Design review of the part shown in the three views and the two pictorial views. Dimensions are in mm from the part's minimum x, y and z. A direction names the side the tool comes from. Give positions to 0.01 mm unless a question says otherwise; leave off trailing zeros. Loops run counter-clockwise (first coordinate to the right, second up) from the corner with the lowest first, then second, coordinate; pieces in that order, holes last. Notation, with made-up numbers: (26.25, 1.25) - (37.25, 1.25) arc R25 ccw to (37.25, 21.25) - close; hole circle Ø7 at (34, 52). An arc over 180 degrees is marked (long way). Answer as a JSON object with one key per item and string values.
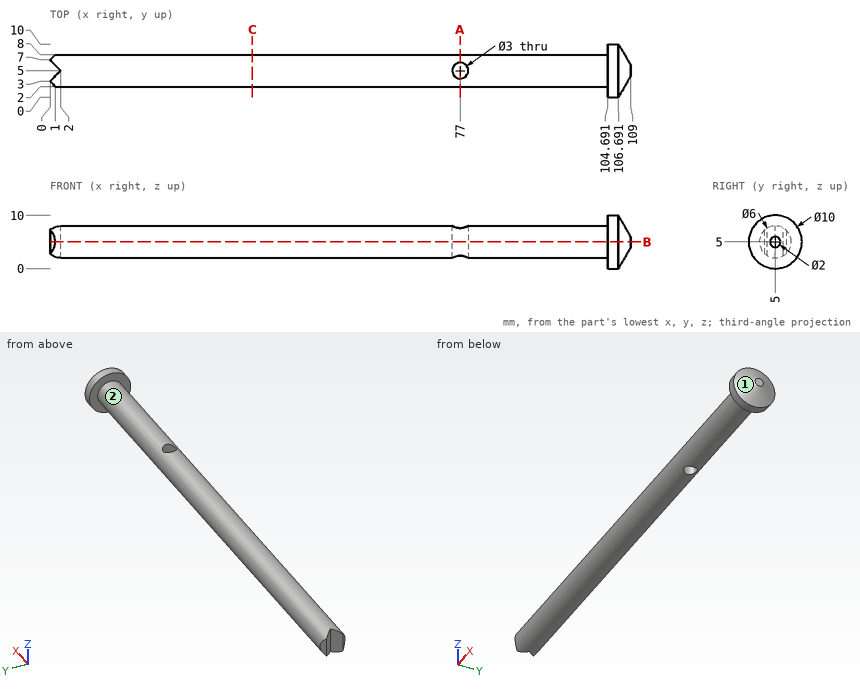
Q1. Clearance check with flat-ended pins moving along their axes: pin 1 Ø3 at (x, y) = (15.5, 8.5) entering from +Z (1 decimal); pin 2 Ø6 at (x, z) = (24, 8) entering from +Y; pin 3 Ø6 at (x, y) = (70, 2) entering from -Z; pin 4 Ø4 at (y, z) = (4, 3) entering from -X. State where each tip first meets the part, or that it passes through.
Results:
{"pin 1": "stops at z = 7.2", "pin 2": "stops at y = 8", "pin 3": "stops at z = 2", "pin 4": "stops at x = 0"}
Q2. Consider section A-A, the plane x = 77. State the section outline as (y, z) points.
Results:
{"outline": "(3.5, 2.4) - (3.5, 7.6) arc R3 ccw to start; (6.5, 2.4) arc R3 ccw to (6.5, 7.6) - close"}
Q3. For the marked faces 1 and 2, list the 3-axis set-ups (+Z, -Z, +X, -X, +Y, -Y) from which the entire face can be reached by the end or side of a thin tool; tool diameter is ignored.
Results:
{"face 1": "+X", "face 2": "-X"}
Q4. Consider section C-C, the plane x = 38. State the section outline as (y, z) points.
Results:
{"outline": "circle Ø6 at (5, 5)"}
Q5. Consider section B-B, the plane z = 5. State the section outline as (x, y) points, plus the area to 3 significant figures.
Results:
{"outline": "(0, 3) - (1, 2) - (104.69, 2) - (104.69, 0) - (106.69, 0) - (109, 4) - (109, 6) - (106.69, 10) - (104.69, 10) - (104.69, 8) - (1, 8) - (0, 7) - (2, 5) - close; hole circle Ø3 at (77, 5)", "area": "650 mm^2"}
Q6. To check wall thickness, follow probe 1 along X at (y, z) = (5, 5); probe 2 along Y at (x, z) = (57, 3) (1 decimal); probe 3 along Y at (x, z) = (77.5, 3.75) (1 decimal). State the ranges of each line that lie inside material, in increasing order. Write a range as [from, to].
Results:
{"probe 1": "x = [2, 75.5], [78.5, 109]", "probe 2": "y = [2.8, 7.2]", "probe 3": "y = [2.3, 3.6], [6.4, 7.7]"}
